```python
from build123d import *

# Parameters (mm, degrees)
SKETCH2_W               = 2
SKETCH2_H               = 80
BOSS_EXTRUDE1_DEPTH     = 6
CONVERT_SOLID1_START    = -6
CONVERT_SOLID1_DEPTH    = 12
CONVERT_SOLID1_2_DEPTH  = 12
CUT_EXTRUDE1_DEPTH      = 81.326747127
CUT_EXTRUDE1_DEPTH_BACK = 81.326747127
SKETCH7_W               = 0.5
SKETCH7_H               = 6


# Read off the part's stored shape, not the designer's step: SharpBend1
with BuildPart() as part:
    # Sketch2 → Boss-Extrude1 (new, symmetric)
    with BuildSketch(Plane(origin=(0, 0, 0), x_dir=(1, 0, 0), z_dir=(0, 1, 0))):
        with Locations((0, 40)):
            Rectangle(SKETCH2_W, SKETCH2_H)
    extrude(amount=BOSS_EXTRUDE1_DEPTH, both=True)

    # Convert-Solid1 outline → Convert-Solid1 (cut)
    with BuildSketch(Plane(origin=(0, 0, 0), x_dir=(1, 0, 0), z_dir=(0, 1, 0)).offset(CONVERT_SOLID1_START)):
        with BuildLine():
            Line((1, 0.5), (1, 80))
            Line((1, 80), (-1, 80))
            Line((-1, 80), (-1, 0.5))
            ThreePointArc((-1, 0.5), (-0.853553391, 0.146446609), (-0.5, 0))
            Line((-0.5, 0), (0.5, 0))
            ThreePointArc((0.5, 0), (0.853553391, 0.146446609), (1, 0.5))
        make_face()
    extrude(amount=CONVERT_SOLID1_DEPTH, mode=Mode.SUBTRACT)

    # Convert-Solid1 2 outline → Convert-Solid1 2 (add)
    with BuildSketch(Plane(origin=(0, 0, 0), x_dir=(1, 0, 0), z_dir=(0, 1, 0)).offset(CONVERT_SOLID1_START)):
        with BuildLine():
            Line((4.048, 0.5), (4.048, 80))
            Line((4.048, 80), (1, 80))
            Line((1, 80), (1, 0))
            Line((1, 0), (-1, 0))
            Line((-1, 0), (-1, 80))
            Line((-1, 80), (-4.048, 80))
            Line((-4.048, 80), (-4.048, 0.5))
            ThreePointArc((-4.048, 0.5), (-3.00881486, -2.00881486), (-0.5, -3.048))
            Line((-0.5, -3.048), (0.5, -3.048))
            ThreePointArc((0.5, -3.048), (3.00881486, -2.00881486), (4.048, 0.5))
        make_face()
    extrude(amount=CONVERT_SOLID1_2_DEPTH)

    # Sketch7 → Cut-Extrude1 (cut, two sides: drawn at the far end of the back side and taken through both)
    with BuildSketch(Plane.XY.offset(-CUT_EXTRUDE1_DEPTH_BACK)):
        with Locations((0, -3)):
            Rectangle(SKETCH7_W, SKETCH7_H)
    extrude(amount=CUT_EXTRUDE1_DEPTH + CUT_EXTRUDE1_DEPTH_BACK, mode=Mode.SUBTRACT)


solid = part.part
```
Here's how the part is built. I have some questions about the finished solid (model axes, mm). A direction names the side the tool comes from. Give positions to 0.01 mm unless a question says otherwise; leave off trailing zeros. Loops run counter-clockwise (first coordinate to the right, second up) from the corner with the lowest first, then second, coordinate; pieces in that order, holes last. Notation, with made-up numbers: M 37.25,82 L 78.25,82 A27 ccw 78.25,114 Z; hole C -21,72.5 d8. An arc over 180 degrees is marked long. Use one line per item in the form item = value. Start each with the question number.
Q1. If we section it at B-B (z = -60): Write out the boundary of the cut face in (x, y), then the cut area to 3 significant figures.
Q2. If we section it at C-C (y = 4.75): Write out the boundary of the cut face in (x, z), then the cut area to 3 significant figures.
Q3. Thinking about a two-plate mould opening in X: for faces 4 (the flat face through (-4.048, 0, -41)), 5 (the flat face through (0.25, -3, 2)), 6 (the cylindrical face through (2.98, -0.08, 2.04)), 7 (the flat face through (-3, 0, -80)), which applies, +X half, -X half, draft (parallel to the pull), parting line (faces both ways), or undercut?
Q4. I need wall thicknesses on line 1 along X through (y, z) = (3, -35.5); line 2 along Z through (x, y) = (-0.5, 2.75); line 3 along Z through (x, y) = (-0.75, -1.5). Which ranges of each line are inside material? Lowest first, please.
Q5. Which directions (+Z, -Z, +X, -X, +Y, -Y) give clear straight access to the entire face, cutting with the end or side of a thin tool? Please do faces 1 (the flat face through (3, 0, -80)), 2 (the flat face through (-0.25, -3, 2)), 3 (the flat face through (1, 0, -41)).
Q6. Will these pins go through, and if not, where does the flat tip stop? pin 1 Ø3 at (x, y) = (-3, 0) entering from +Z; pin 2 Ø2.5 at (y, z) = (-2, 2) entering from -X; pin 3 Ø1.5 at (y, z) = (-3.5, 2) entering from +X.
Q7. If we section it at A-A (y = -2.5): Write out the boundary of the cut face in (x, z).
Taken from the geometry:
q1.outline = M -4.05,-6 L -1,-6 L -1,6 L -4.05,6 Z; M 1,-6 L 4.05,-6 L 4.05,6 L 1,6 Z
q1.area = 73.2 mm^2
q2.outline = M -4.05,-80 L -1,-80 L -1,-0.5 A0.5 cw -0.5,0 L 0.5,0 A0.5 cw 1,-0.5 L 1,-80 L 4.05,-80 L 4.05,-0.5 A3.55 ccw 0.5,3.05 L -0.5,3.05 A3.55 ccw -4.05,-0.5 Z
q2.area = 507 mm^2
q3.face_4 = -X half
q3.face_5 = undercut
q3.face_6 = +X half
q3.face_7 = draft
q4.line_1 = -4.05 to -1, 1 to 4.05
q4.line_2 = 0 to 3.05
q4.line_3 = -0.07 to 3.04
q5.face_1 = -Z, +X, -X, +Y, -Y
q5.face_2 = +Z, -Z, -Y
q5.face_3 = -Z, +Y, -Y
q6.pin_1 = 2.9
q6.pin_2 = -3.82
q6.pin_3 = 3.59
q7.outline = M -4.05,-80 L -1,-80 L -1,-0.5 A0.5 cw -0.5,0 L -0.25,0 L -0.25,3.05 L -0.5,3.05 A3.55 ccw -4.05,-0.5 Z; M 0.25,0 L 0.5,0 A0.5 cw 1,-0.5 L 1,-80 L 4.05,-80 L 4.05,-0.5 A3.55 ccw 0.5,3.05 L 0.25,3.05 Z
